Source: CAD feature listing. Evaluate the final solid. Frame: model axes, mm. Face numbers are marked on the shaded views. A direction names the side the tool comes from. Round coordinates to 2 decimals unless told otherwise and drop trailing zeros. Write each loop counter-clockwise with the first axis right and the second up, starting at its lowest first coordinate (ties: lowest second). Pieces come first, ordered by that corner, then holes.
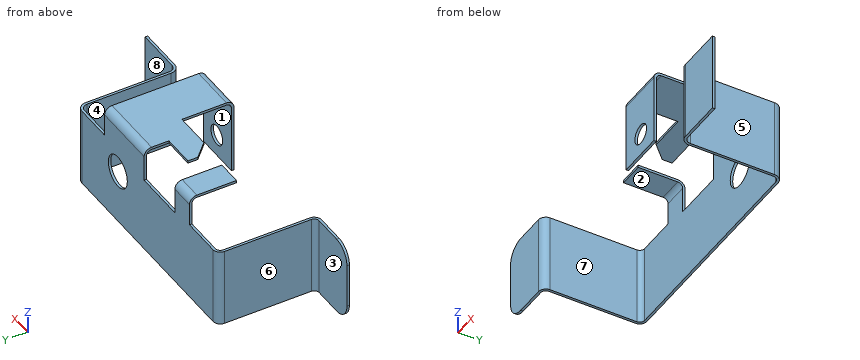
from build123d import *

# Parameters (mm, degrees)
BASE_FLANGE1_DEPTH           = 1
EDGE_FLANGE2_STRIP_W         = 8
EDGE_FLANGE2_STRIP_H         = 1
EDGE_FLANGE2_STRIP_CUT_DEPTH = 32
EDGE_FLANGE2_DEPTH           = 32
EDGE_FLANGE3_STRIP_W         = 8
EDGE_FLANGE3_STRIP_H         = 1
EDGE_FLANGE3_STRIP_CUT_DEPTH = 32
EDGE_FLANGE3_DEPTH           = 32
BASE_FLANGE2_DEPTH           = 10
SKETCH28_W                   = 30.5
SKETCH28_H                   = 1
BASE_FLANGE3_DEPTH           = 21
BASE_FLANGE4_DEPTH           = 8
TAB1_DEPTH                   = 1
BASE_FLANGE5_DEPTH           = 19
SKETCH41_W                   = 32
SKETCH41_H                   = 1
BASE_FLANGE6_DEPTH           = 19
EDGE_FLANGE4_STRIP_W         = 9
EDGE_FLANGE4_STRIP_H         = 1
EDGE_FLANGE4_STRIP_CUT_DEPTH = 32
EDGE_FLANGE4_DEPTH           = 32
EDGE_FLANGE5_STRIP_W         = 9
EDGE_FLANGE5_STRIP_H         = 1
EDGE_FLANGE5_STRIP_CUT_DEPTH = 32
EDGE_FLANGE5_DEPTH           = 32
SKETCH52_R                   = 6.482448702
CUT_EXTRUDE1_DEPTH           = 10
SKETCH53_R                   = 4
CUT_EXTRUDE2_DEPTH           = 10


# Read off the part's stored shape, not the designer's step: Base-Flange2
# Sheet-metal steps are written as plain solids
with BuildPart() as part:
    # Sketch1 → Base-Flange1 (new body)
    with BuildSketch(Plane(origin=(0, 0, 0), x_dir=(1, 0, 0), z_dir=(0, 1, 0))):
        with BuildLine():
            Line((-33.194191811, -9), (-33.194191811, 9))
            ThreePointArc((-33.194191811, 9), (-31.14393928, 13.949747468), (-26.194191811, 16))
            Line((-26.194191811, 16), (-11.194191811, 16))
            Line((-11.194191811, 16), (-11.194191811, -16))
            Line((-11.194191811, -16), (-26.194191811, -16))
            ThreePointArc((-26.194191811, -16), (-31.14393928, -13.949747468), (-33.194191811, -9))
        make_face()
    extrude(amount=-BASE_FLANGE1_DEPTH)

    # Edge-Flange2 strip (across the edge) → Edge-Flange2 strip cut (cut)
    with BuildSketch(Plane(origin=(-11.194191811, 0, 16), x_dir=(-1, 0, 0), z_dir=(0, 0, -1))):
        with Locations((-1, -0.5)):
            Rectangle(EDGE_FLANGE2_STRIP_W, EDGE_FLANGE2_STRIP_H)
    extrude(amount=EDGE_FLANGE2_STRIP_CUT_DEPTH, mode=Mode.SUBTRACT)

    # Edge-Flange2 section (across the edge) → Edge-Flange2 (add)
    with BuildSketch(Plane(origin=(-11.194191811, 0, 16), x_dir=(-1, 0, 0), z_dir=(0, 0, -1))):
        with BuildLine():
            Line((0, 2), (0, 40))
            Line((0, 40), (1, 40))
            Line((1, 40), (1, 2))
            ThreePointArc((1, 2), (1.585786438, 0.585786438), (3, 0))
            Line((3, 0), (3, -1))
            ThreePointArc((3, -1), (0.878679656, -0.121320344), (0, 2))
        make_face()
    extrude(amount=EDGE_FLANGE2_DEPTH)

    # Edge-Flange3 strip (across the edge) → Edge-Flange3 strip cut (cut)
    with BuildSketch(Plane(origin=(-11.194191811, 40, -16), x_dir=(0, -1, 0), z_dir=(0, 0, 1))):
        with Locations((-1, -0.5)):
            Rectangle(EDGE_FLANGE3_STRIP_W, EDGE_FLANGE3_STRIP_H)
    extrude(amount=EDGE_FLANGE3_STRIP_CUT_DEPTH, mode=Mode.SUBTRACT)

    # Edge-Flange3 section (across the edge) → Edge-Flange3 (add)
    with BuildSketch(Plane(origin=(-11.194191811, 40, -16), x_dir=(0, -1, 0), z_dir=(0, 0, 1))):
        with BuildLine():
            Line((0, 2), (0, 18))
            Line((0, 18), (1, 18))
            Line((1, 18), (1, 2))
            ThreePointArc((1, 2), (1.585786438, 0.585786438), (3, 0))
            Line((3, 0), (3, -1))
            ThreePointArc((3, -1), (0.878679656, -0.121320344), (0, 2))
        make_face()
    extrude(amount=EDGE_FLANGE3_DEPTH)


with BuildPart() as body_2:
    # Base-Flange2 outline → Base-Flange2 (new body)
    with BuildSketch(Plane(origin=(6.805808189, 0, 0), x_dir=(0, 0, -1), z_dir=(1, 0, 0))):
        with BuildLine():
            Line((-28, 37), (-28, 21))
            Line((-28, 21), (-27, 21))
            Line((-27, 21), (-27, 37))
            ThreePointArc((-27, 37), (-26.414213562, 38.414213562), (-25, 39))
            Line((-25, 39), (16, 39))
            Line((16, 39), (16, 40))
            Line((16, 40), (-25, 40))
            ThreePointArc((-25, 40), (-27.121320344, 39.121320344), (-28, 37))
        make_face()
    extrude(amount=BASE_FLANGE2_DEPTH)


with BuildPart() as part_1:
    add(part.part)

    # Combine1: union body 2
    add(body_2.part)


with BuildPart() as body_2_2:
    # Sketch28 → Base-Flange3 (new body)
    with BuildSketch(Plane(origin=(16.805808189, 0, 0), x_dir=(0, 0, -1), z_dir=(1, 0, 0))):
        with Locations((0.75, 39.5)):
            Rectangle(SKETCH28_W, SKETCH28_H)
    extrude(amount=BASE_FLANGE3_DEPTH)


with BuildPart() as body_3:
    # Sketch31 → Base-Flange4 (new body)
    with BuildSketch(Plane(origin=(37.805808189, 0, 0), x_dir=(0, 0, -1), z_dir=(1, 0, 0))):
        with BuildLine():
            Line((16, 39), (-25, 39))
            ThreePointArc((-25, 39), (-26.414213562, 38.414213562), (-27, 37))
            Line((-27, 37), (-27, 30))
            Line((-27, 30), (-28, 30))
            Line((-28, 30), (-28, 37))
            ThreePointArc((-28, 37), (-27.121320344, 39.121320344), (-25, 40))
            Line((-25, 40), (16, 40))
            Line((16, 40), (16, 39))
        make_face()
    extrude(amount=BASE_FLANGE4_DEPTH)

    # Sketch34 → Tab1 (add)
    with BuildSketch(Plane.XY.offset(28)):
        Polygon((45.805808189, 30), (24.805808189, 30), (24.805808189, 26), (30.805808189, 20), (45.805808189, 20), align=None)
    extrude(amount=-TAB1_DEPTH)


with BuildPart() as body_4:
    # Sketch38 → Base-Flange5 (new body)
    with BuildSketch(Plane(origin=(45.805808189, 0, 0), x_dir=(0, 0, -1), z_dir=(1, 0, 0))):
        with BuildLine():
            Line((16, 39), (-25, 39))
            ThreePointArc((-25, 39), (-26.414213562, 38.414213562), (-27, 37))
            Line((-27, 37), (-27, 2))
            ThreePointArc((-27, 2), (-26.414213562, 0.585786438), (-25, 0))
            Line((-25, 0), (3, 0))
            Line((3, 0), (3, -1))
            Line((3, -1), (-25, -1))
            ThreePointArc((-25, -1), (-27.121320344, -0.121320344), (-28, 2))
            Line((-28, 2), (-28, 37))
            ThreePointArc((-28, 37), (-27.121320344, 39.121320344), (-25, 40))
            Line((-25, 40), (16, 40))
            Line((16, 40), (16, 39))
        make_face()
    extrude(amount=BASE_FLANGE5_DEPTH)


with BuildPart() as body_5:
    # Sketch41 → Base-Flange6 (new body)
    with BuildSketch(Plane(origin=(64.805808189, 0, 0), x_dir=(0, 0, -1), z_dir=(1, 0, 0))):
        with Locations((0, 39.5)):
            Rectangle(SKETCH41_W, SKETCH41_H)
    extrude(amount=BASE_FLANGE6_DEPTH)

    # Edge-Flange4 strip (across the edge) → Edge-Flange4 strip cut (cut)
    with BuildSketch(Plane(origin=(83.805808189, 39, -16), x_dir=(-1, 0, 0), z_dir=(0, 0, 1))):
        with Locations((-1, -0.5)):
            Rectangle(EDGE_FLANGE4_STRIP_W, EDGE_FLANGE4_STRIP_H)
    extrude(amount=EDGE_FLANGE4_STRIP_CUT_DEPTH, mode=Mode.SUBTRACT)

    # Edge-Flange4 section (across the edge) → Edge-Flange4 (add)
    with BuildSketch(Plane(origin=(83.805808189, 39, -16), x_dir=(-1, 0, 0), z_dir=(0, 0, 1))):
        with BuildLine():
            Line((0, 2.5), (0, 40))
            Line((0, 40), (1, 40))
            Line((1, 40), (1, 2.5))
            ThreePointArc((1, 2.5), (1.732233047, 0.732233047), (3.5, 0))
            Line((3.5, 0), (3.5, -1))
            ThreePointArc((3.5, -1), (1.025126266, 0.025126266), (0, 2.5))
        make_face()
    extrude(amount=EDGE_FLANGE4_DEPTH)

    # Edge-Flange5 strip (across the edge) → Edge-Flange5 strip cut (cut)
    with BuildSketch(Plane(origin=(83.805808189, -1, 16), x_dir=(0, 1, 0), z_dir=(0, 0, -1))):
        with Locations((-1, -0.5)):
            Rectangle(EDGE_FLANGE5_STRIP_W, EDGE_FLANGE5_STRIP_H)
    extrude(amount=EDGE_FLANGE5_STRIP_CUT_DEPTH, mode=Mode.SUBTRACT)

    # Edge-Flange5 section (across the edge) → Edge-Flange5 (add)
    with BuildSketch(Plane(origin=(83.805808189, -1, 16), x_dir=(0, 1, 0), z_dir=(0, 0, -1))):
        with BuildLine():
            Line((0, 2.5), (0, 21))
            Line((0, 21), (1, 21))
            Line((1, 21), (1, 2.5))
            ThreePointArc((1, 2.5), (1.732233047, 0.732233047), (3.5, 0))
            Line((3.5, 0), (3.5, -1))
            ThreePointArc((3.5, -1), (1.025126266, 0.025126266), (0, 2.5))
        make_face()
    extrude(amount=EDGE_FLANGE5_DEPTH)


with BuildPart() as body_2_2_1:
    add(body_2_2.part)

    # Combine2: union body 3, body 4, body 5, part
    add(body_3.part)
    add(body_4.part)
    add(body_5.part)
    add(part_1.part)

    # Sketch52 → Cut-Extrude1 (cut)
    with BuildSketch(Plane(origin=(0, 40, 0), x_dir=(1, 0, 0), z_dir=(0, 1, 0))):
        with Locations(Location((55.805808189, -6, 0), (0, 0, 270))):
            Circle(SKETCH52_R)
    extrude(amount=-CUT_EXTRUDE1_DEPTH, mode=Mode.SUBTRACT)

    # Sketch53 → Cut-Extrude2 (cut)
    with BuildSketch(Plane(origin=(0, 0, 0), x_dir=(1, 0, 0), z_dir=(0, 1, 0))):
        with Locations(Location((55.805808189, -6, 0), (0, 0, 270))):
            Circle(SKETCH53_R)
    extrude(amount=-CUT_EXTRUDE2_DEPTH, mode=Mode.SUBTRACT)


solid = body_2_2_1.part
1) Reachability of the marked faces 1, 2, 3, 4 and 5 from +Z, -Z, +X, -X, +Y, -Y: full face, straight path, thin tool, end or side. Return the list, or none.
Taken from the geometry:
face 1: -Z
face 2: -Z, +X, -X, -Y
face 3: +Z, -Z, -X, +Y
face 4: +Z, -Z, -Y
face 5: +Z, -Z, +X, +Y
2) Material intervals for line 1 (X direction, y = 26.5, z = 4); line 2 (Y direction, x = 55, z = 14.5); line 3 (Y direction, x = 40, z = 3), sorted ascending.
Taken from the geometry:
line 1: x = -12.19 to -11.19, 82.81 to 83.81
line 2: y = -1 to 0, 39 to 40
line 3: y = 39 to 40
3) Pull-direction query (X, two-part tool) for the marked faces 6, 7 and 8; classes: released by +X, released by -X, zero draft, split by the parting line, or undercut.
Taken from the geometry:
face 6: released by -X
face 7: undercut
face 8: zero draft
4) Section query D-D on y = 14.5. Return the cut outline in (x, z), then the cut area to 3 significant figures.
Taken from the geometry:
outline: (-12.19, -16) - (-11.19, -16) - (-11.19, 16) - (-12.19, 16) - close; (45.81, 27) - (64.81, 27) - (64.81, 28) - (45.81, 28) - close; (82.81, -16) - (83.81, -16) - (83.81, 16) - (82.81, 16) - close
area: 83.0 mm2
5) Contact query for flat-ended pins moving along their axis: P1, Ø10, axis at y = 10, z = 17.5, coming from the +X side; P2, Ø10.5, axis at y = 9.5, z = 13.5, coming from the -X side; P3, Ø9, axis at x = 96.5, z = -5.5, coming from the +Y side. Output: stop coordinate, or through.
Taken from the geometry:
P1: stops at x = 83.81
P2: stops at x = -12.19
P3: stops at y = 0
6) Section query B-B on z = 20. Return the cut outline in (x, y), then the cut area to 3 significant figures.
Taken from the geometry:
outline: (6.81, 39) - (16.81, 39) - (16.81, 40) - (6.81, 40) - close; (37.81, 39) - (64.81, 39) - (64.81, 40) - (37.81, 40) - close; (45.81, -1) - (64.81, -1) - (64.81, 0) - (45.81, 0) - close
area: 56.0 mm2
7) Section query C-C on x = 29. Return the cut outline in (y, z).
Taken from the geometry:
outline: (21.81, 27) - (30, 27) - (30, 28) - (21.81, 28) - close; (39, -16) - (40, -16) - (40, 14.5) - (39, 14.5) - close
8) Section query A-A on y = 27.5. Return the cut outline in (x, z).
Taken from the geometry:
outline: (-12.19, -16) - (-11.19, -16) - (-11.19, 16) - (-12.19, 16) - close; (6.81, 27) - (16.81, 27) - (16.81, 28) - (6.81, 28) - close; (24.81, 27) - (64.81, 27) - (64.81, 28) - (24.81, 28) - close; (82.81, -16) - (83.81, -16) - (83.81, 16) - (82.81, 16) - close
